Geometry: see drawing. Coordinates: mm, zero at the bounding-box minimum. A direction names the side the tool comes from. Coordinates: 2 decimals unless noted, no trailing zeros. Write each loop counter-clockwise with the first axis right and the second up, starting at its lowest first coordinate (ties: lowest second). Pieces come first, ordered by that corner, then holes.
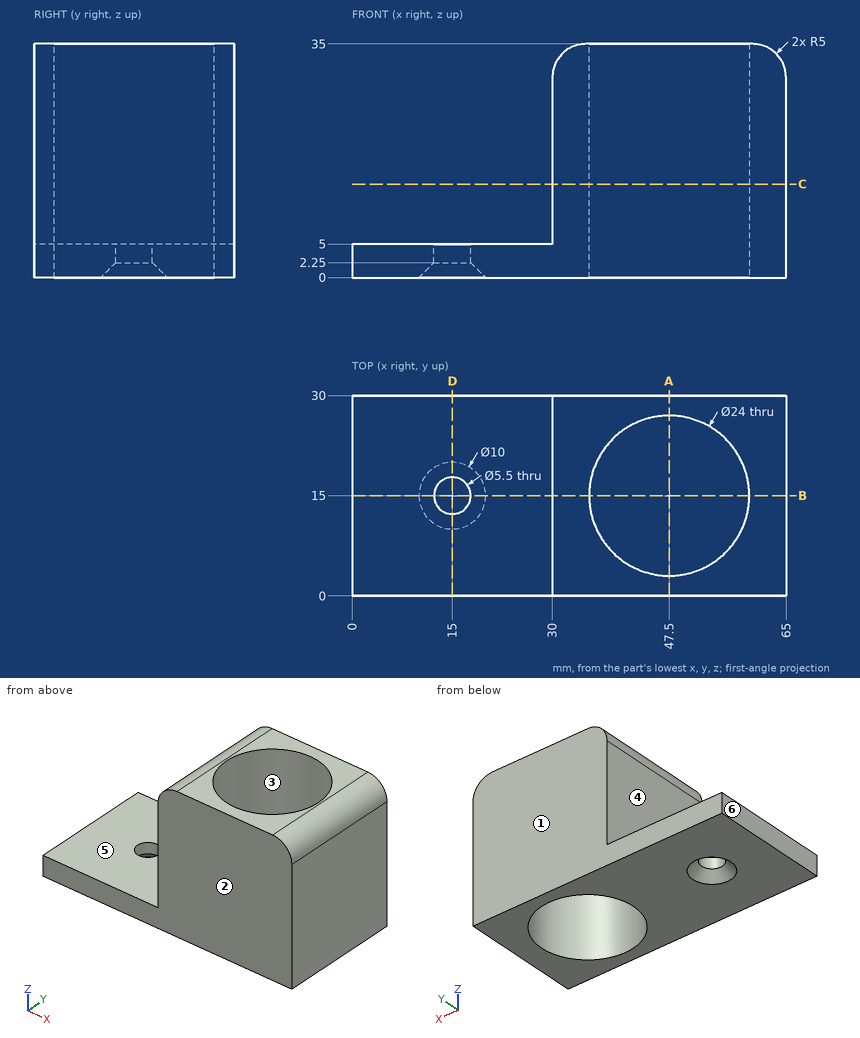
Item 1: Pin query (flat end, axial travel): pin 1 (8 mm diameter, centred on y = 8, z = 23.5, fed in from -X); pin 2 (9 mm diameter, centred on x = 15.5, y = 19, fed in from +Z). Return the tip coordinate at first contact, or that it passes through.
Derived:
pin 1: stops at x = 30
pin 2: stops at z = 5
Item 2: Section D-D, the plane x = 15. Output: boundary loops of the cut face in (y, z).
Derived:
outline: (0, 0) - (10, 0) - (12.25, 2.25) - (12.25, 5) - (0, 5) - close; (17.75, 2.25) - (20, 0) - (30, 0) - (30, 5) - (17.75, 5) - close
Item 3: Section B-B, the plane y = 15. Output: boundary loops of the cut face in (x, z), plus the area to 3 significant figures.
Derived:
outline: (0, 0) - (10, 0) - (12.25, 2.25) - (12.25, 5) - (0, 5) - close; (17.75, 2.25) - (20, 0) - (35.5, 0) - (35.5, 35) - (35, 35) arc R5 ccw to (30, 30) - (30, 5) - (17.75, 5) - close; (59.5, 0) - (65, 0) - (65, 30) arc R5 ccw to (60, 35) - (59.5, 35) - close
area: 492 mm2
Item 4: Pull-direction query (Y, two-part tool) for the marked faces 1, 2, 3 and 4; classes: released by +Y, released by -Y, zero draft, split by the parting line, or undercut.
Derived:
face 1: released by +Y
face 2: released by -Y
face 3: undercut
face 4: zero draft
Item 5: Section C-C, the plane z = 14. Output: boundary loops of the cut face in (x, y), plus the area to 3 significant figures.
Derived:
outline: (30, 0) - (65, 0) - (65, 30) - (30, 30) - close; hole circle Ø24 at (47.5, 15)
area: 598 mm2
Item 6: Set-up query: the marked faces 5 and 6. Return all of +Z, -Z, +X, -X, +Y, -Y with unobstructed straight access to the full face (end or side cutting, diameter ignored); none if empty.
Derived:
face 5: +Z, -X, +Y, -Y
face 6: +Z, -Z, -X, +Y, -Y
Item 7: Section A-A, the plane x = 47.5. Output: boundary loops of the cut face in (y, z), plus the area to 3 significant figures.
Derived:
outline: (0, 0) - (3, 0) - (3, 35) - (0, 35) - close; (27, 0) - (30, 0) - (30, 35) - (27, 35) - close
area: 210 mm2
Item 8: Material intervals for probe 1 along Y at (x, z) = (15, 4); probe 2 along Y at (x, z) = (47.5, 28.5); probe 3 along X at (y, z) = (12.5, 2), sorted ascending.
Derived:
probe 1: y = 0 to 12.25, 17.75 to 30
probe 2: y = 0 to 3, 27 to 30
probe 3: x = 0 to 13.34, 16.66 to 35.76, 59.24 to 65
